Drawing for the job (mm, zero at the part's lowest x, y, z). Round coordinates to 2 decimals unless told otherwise and drop trailing zeros. Write each loop counter-clockwise with the first axis right and the second up, starting at its lowest first coordinate (ties: lowest second). Pieces come first, ordered by that corner, then holes.
Item 1: Band-saw the part on A-A, the plane x = 9.5. Write the cut outline in (y, z), then the cut area to 3 significant figures.
Item 2: Band-saw the part on B-B, the plane y = 8. Write the cut outline in (x, z).
Item 3: Band-saw the part on D-D, the plane z = 1.15. Count the separate pieces of the cut face and the enclosed holes in it.
Item 4: Wall check: probe 1 along Y at (x, z) = (9.5, 0.6); probe 2 along Y at (x, z) = (8.25, 0.2); probe 3 along X at (y, z) = (12, 0.4) (1 decimal). Give the ranges that are in metal, low to high.
Item 5: Band-saw the part on C-C, the plane y = 14. Write the cut outline in (x, z).
Item 6: Mould opens along Y. For the marked faces 1, 2, 3 and 4 say: +Y half, -Y half, draft (parallel to the pull), parting line (faces both ways), or undercut.
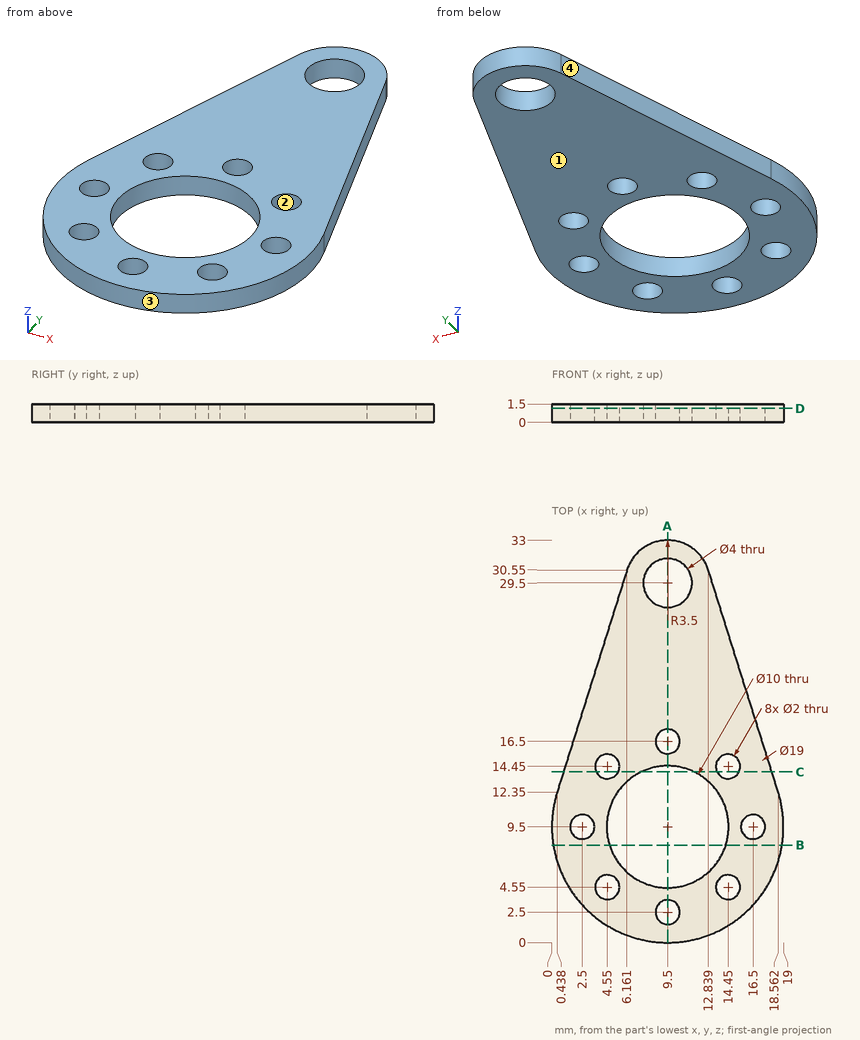
Results:
1. outline: (0, 0) - (1.5, 0) - (1.5, 1.5) - (0, 1.5) - close; (3.5, 0) - (4.5, 0) - (4.5, 1.5) - (3.5, 1.5) - close; (14.5, 0) - (15.5, 0) - (15.5, 1.5) - (14.5, 1.5) - close; (17.5, 0) - (27.5, 0) - (27.5, 1.5) - (17.5, 1.5) - close; (31.5, 0) - (33, 0) - (33, 1.5) - (31.5, 1.5) - close
1. area: 22.5 mm2
2. outline: (0.12, 0) - (4.73, 0) - (4.73, 1.5) - (0.12, 1.5) - close; (14.27, 0) - (18.88, 0) - (18.88, 1.5) - (14.27, 1.5) - close
3. separate pieces: 1
3. enclosed holes: 10
4. probe 1: y = 0 to 1.5, 3.5 to 4.5, 14.5 to 15.5, 17.5 to 27.5, 31.5 to 33
4. probe 2: y = 0.08 to 4.66, 14.34 to 27.94, 31.06 to 32.77
4. probe 3: x = 0.3 to 5.2, 13.8 to 18.7
5. outline: (0.96, 0) - (3.66, 0) - (3.66, 1.5) - (0.96, 1.5) - close; (5.44, 0) - (7.32, 0) - (7.32, 1.5) - (5.44, 1.5) - close; (11.68, 0) - (13.56, 0) - (13.56, 1.5) - (11.68, 1.5) - close; (15.34, 0) - (18.04, 0) - (18.04, 1.5) - (15.34, 1.5) - close
6. face 1: draft
6. face 2: undercut
6. face 3: parting line
6. face 4: +Y half
